Job drawing, mm, ordinate dimensions from the low corner. One solid piece. Coordinates: 2 decimals unless noted, no trailing zeros. Write each loop counter-clockwise with the first axis right and the second up, starting at its lowest first coordinate (ties: lowest second). Pieces come first, ordered by that corner, then holes. Notation, with made-up numbers: (31, 0) - (73, 0) arc R12 cw to (73, 8) - close; hole circle Ø7 at (-38.5, 31). An arc over 180 degrees is marked (long way). Put each result on its own line as item: value. Start each with the question number.
1. Saw through at A-A, the plane x = 4.5. Write the cut outline in (y, z), plus the area to 3 significant figures.
2. Pull direction X, two halves, no side cores. Call the marked faces 1, 2, 3 and 4: released by +X, released by -X, zero draft, split by the parting line, or undercut.
3. Saw through at B-B, the plane z = 2.45. Write the cut outline in (x, y), plus the area to 3 significant figures.
4. Drop flat-ended pins along their axis: P1, Ø1.5, axis at x = 1.5, z = 1.5, coming from the -Y side; P2, Ø1, axis at y = 1, z = 1.5, coming from the -X side; P3, Ø1, axis at x = 7.5, z = 2, coming from the -Y side. Give the stop position or say it passes through.
5. Drill centre lines: L1, parallel to X at y = 4.5, z = 0.3; L2, parallel to X at y = 4.5, z = 1.6. Where is each one in solid material? Low to high. Write a range as from..to.
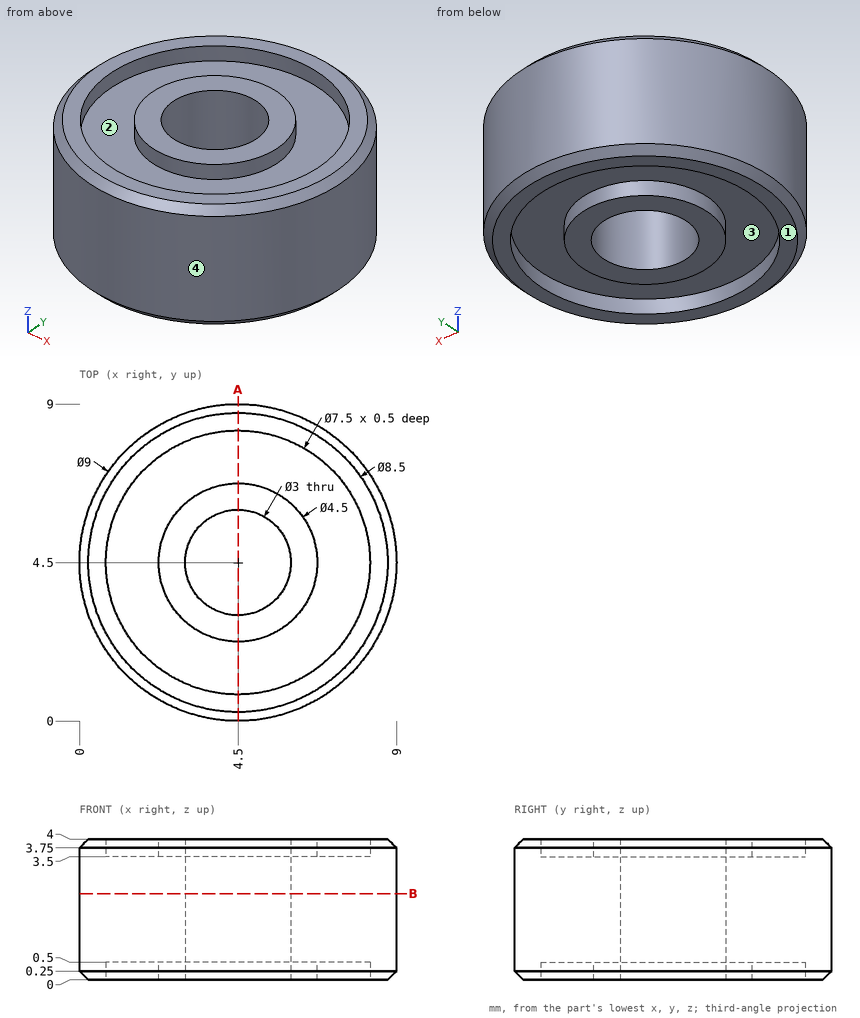
Final values:
1. outline: (0, 0.25) - (0.25, 0) - (0.75, 0) - (0.75, 0.5) - (2.25, 0.5) - (2.25, 0) - (3, 0) - (3, 4) - (2.25, 4) - (2.25, 3.5) - (0.75, 3.5) - (0.75, 4) - (0.25, 4) - (0, 3.75) - close; (6, 0) - (6.75, 0) - (6.75, 0.5) - (8.25, 0.5) - (8.25, 0) - (8.75, 0) - (9, 0.25) - (9, 3.75) - (8.75, 4) - (8.25, 4) - (8.25, 3.5) - (6.75, 3.5) - (6.75, 4) - (6, 4) - close
1. area: 20.9 mm²
2. face 1: zero draft
2. face 2: undercut
2. face 3: undercut
2. face 4: split by the parting line
3. outline: circle Ø9 at (4.5, 4.5); hole circle Ø3 at (4.5, 4.5)
3. area: 56.5 mm²
4. P1: stops at y = 0.6
4. P2: stops at x = 1.15
4. P3: stops at y = 0.76
5. L1: x = 0..0.75, 2.25..3, 6..6.75, 8.25..9
5. L2: x = 0..3, 6..9
